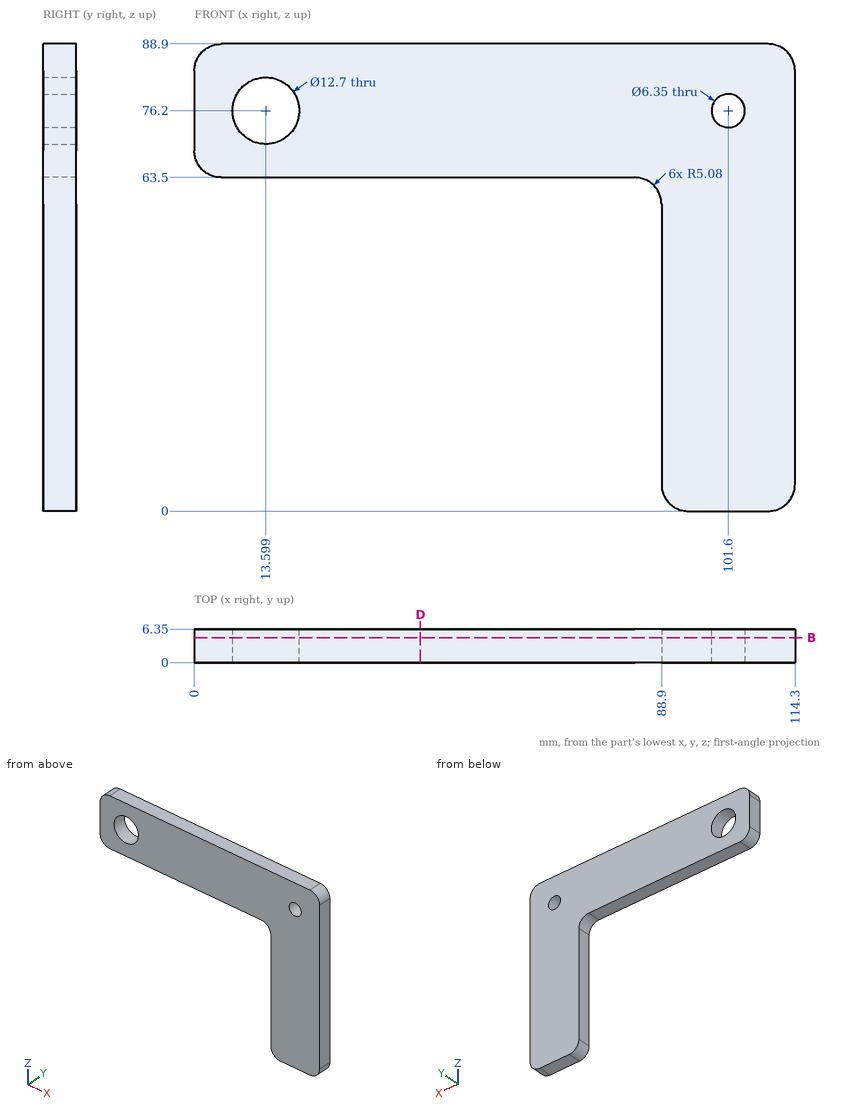
The figure shows three views and two pictorial views of one solid part (mm, origin at its lowest corner). Answer the questions. Round coordinates to 2 decimals unless told otherwise and drop trailing zeros. Order: outer loops, then holes, each group sorted by start corner. A loop starts at its lowest first (then second) coordinate and runs counter-clockwise, first axis right, second up.
Q1. Find the intervals of material crossed by line 1 along Z through (x, y) = (101.6, 3.75) (1 decimal); line 2 along X through (y, z) = (1, 32.5); line 3 along Z through (x, y) = (44, 5.75), in increasing order.
Solution:
line 1: z = 0 to 73, 79.4 to 88.9
line 2: x = 88.9 to 114.3
line 3: z = 63.5 to 88.9
Q2. A cutting plane is placed at B-B, the plane y = 4.75. Count the separate pieces of the cut face and the enclosed holes in it, then the cut area to 3 significant figures.
Solution:
separate pieces: 1
enclosed holes: 2
area: 4,340 mm2
Q3. A cutting plane is placed at D-D, the plane x = 43. Determine the outline of the cut face in (y, z), then the cut area to 3 significant figures.
Solution:
outline: (0, 63.5) - (6.35, 63.5) - (6.35, 88.9) - (0, 88.9) - close
area: 161 mm2
